```python
from build123d import *

# Parameters (mm, degrees)
F1_DEPTH = 11
F2_D     = 6.3
F3_R     = 5
F4_R     = 2
F5_R     = 1


with BuildPart() as f1:
    # F0 (on Front) → F1 (new body)
    with BuildSketch(Plane.XZ):
        with BuildLine():
            Line((19.1313266688, -1.3), (-19.6425261418, -1.3))
            ThreePointArc((-19.6425261418, -1.3), (-20.5226323435, 3.3504941743), (-24.5, 5.9160797831))
            Line((-24.5, 5.9160797831), (-24.5, 11.5))
            Line((-24.5, 11.5), (-37.5, 11.5))
            Line((-37.5, 11.5), (-37.5, 3.730095943))
            Line((-37.5, 3.730095943), (-26.5, -5.5))
            Line((-26.5, -5.5), (26.5, -5.5))
            ThreePointArc((26.5, -5.5), (37.7208276523, 1.8760988126), (50.5, 6))
            Line((50.5, 6), (50.5, 11.5))
            Line((50.5, 11.5), (38.5, 11.5))
            Line((38.5, 11.5), (28.5361144551, 5.7473479985))
            ThreePointArc((28.5361144551, 5.7473479985), (21.6022101623, 5.2016568881), (19.1313266688, -1.3))
        make_face()
    extrude(amount=-F1_DEPTH)

    # F2 (through all)
    with Locations(Plane.XZ):
        with Locations((25.5, 0), (-25.5, 0)):
            Hole(F2_D / 2)

    # F3
    f3_edges = [f1.edges().sort_by_distance(p)[0] for p in [
        (-24.5, 5.5, 5.91608),
        (-19.642526, 5.5, -1.3),
        (19.131327, 5.5, -1.3),
        (28.536114, 5.5, 5.747348),
        (-37.5, 5.5, 3.730096),
        (-26.5, 5.5, -5.5),
        (26.5, 5.5, -5.5),
        (38.5, 5.5, 11.5),
    ]]
    fillet(f3_edges, radius=F3_R)

    # F4
    f4_edges = [f1.edges().sort_by_distance(p)[0] for p in [
        (-24.5, 5.5, 11.5),
        (-37.5, 5.5, 11.5),
        (50.5, 5.5, 11.5),
        (50.5, 5.5, 6),
    ]]
    fillet(f4_edges, radius=F4_R)

    # F5
    f5_edges = [f1.edges().sort_by_distance(p)[0] for p in [
        (28.771496, 11, 6.278411),
        (-0.264736, 0, -1.3),
    ]]
    fillet(f5_edges, radius=F5_R)


solid = f1.part
```
Geometry check sheet. Reference: the model listing, model coordinates, mm. A direction names the side the tool comes from. Coordinates: 2 decimals unless noted, no trailing zeros. Loops run counter-clockwise (first coordinate to the right, second up) from the corner with the lowest first, then second, coordinate; pieces in that order, holes last. Notation, with made-up numbers: (60.25, -17) - (102.25, -17) arc R15 cw to (102.25, 6) - close; hole circle Ø7 at (44.5, 64.25). An arc over 180 degrees is marked (long way). One line per item, written item: value. Start each with the question number.
(1) Cross-section at B-B on z = 0. Count the separate pieces of the cut face and the enclosed holes in it, plus the area to 3 significant figures.
(2) Mould release check, pull along Z, two halves, no side actions. Record for faces 4 (the cylindrical face through (38.528, 5.563, 11.325)), 5 (the cylindrical face through (22.59, 5.58, -1.21)), 6 (the cylindrical face through (-31.675, 10.699, -0.785)): released by +Z, released by -Z, zero draft, split by the parting line, or undercut.
(3) Material ranges on line 1 (Z direction, x = -6, y = 9); line 2 (X direction, y = 2.25, z = 9); line 3 (Z direction, x = -25.5, y = 3.5), recorded low to high. Write a range as [from, to].
(4) Depth check by flat-ended pin: P1, Ø1.5, axis at x = 33, y = 4.5, coming from the -Z side; P2, Ø10, axis at x = 25.5, z = 0, coming from the -Y side; P3, Ø1.5, axis at y = 5.5, z = 1, coming from the -X side; P4, Ø1, axis at x = 35.5, y = 4, coming from the -Z side. Enter the tip coordinate at first touch or a pass-through.
(5) Cross-section at A-A on y = 2.25. Enter the section's corners in (x, z), plus the area to 3 significant figures.
(6) Tool access check on faces 1 (the cylindrical face through (-23.88, 5.56, 6.81)), 2 (the flat face through (-37.5, 5, 8)), 3 (the cylindrical face through (34.031, 0.285, 8.573)). Record the directions out of +Z, -Z, +X, -X, +Y, -Y that give a thin tool (end or side, any length) a straight path to the whole face; none if there is none.
Results below:
1. separate pieces: 4
1. enclosed holes: 0
1. area: 197 mm2
2. face 4: released by +Z
2. face 5: undercut
2. face 6: released by -Z
3. line 1: z = [-5.5, -1.3]
3. line 2: x = [-37.5, -24.5], [34.17, 50.5]
3. line 3: z = [-5.43, -3.15], [3.15, 11.23]
4. P1: stops at z = -1.18
4. P2: stops at y = 0
4. P3: stops at x = -35.14
4. P4: stops at z = 0.47
5. outline: (-37.5, 6.06) arc R5 ccw to (-35.71, 2.23) - (-27.89, -4.33) arc R5 ccw to (-24.68, -5.5) - (24.68, -5.5) arc R5 ccw to (27.83, -4.38) arc R50 cw to (48.92, 5.69) arc R2 ccw to (50.5, 7.65) - (50.5, 9.5) arc R2 ccw to (48.5, 11.5) - (39.84, 11.5) arc R5 ccw to (37.34, 10.83) - (30.52, 6.89) arc R5 cw to (26.92, 6.34) arc R6.5 ccw to (19.35, 2.09) arc R5 cw to (14.61, -1.3) - (-15.14, -1.3) arc R5 cw to (-19.85, 2.02) arc R6 ccw to (-22.23, 5.03) arc R5 cw to (-24.5, 9.22) - (-24.5, 9.5) arc R2 ccw to (-26.5, 11.5) - (-35.5, 11.5) arc R2 ccw to (-37.5, 9.5) - close; hole circle Ø6.3 at (-25.5, 0); hole circle Ø6.3 at (25.5, 0)
5. area: 603 mm2
6. face 1: +Z, +Y, -Y
6. face 2: +Z, -Z, -X, +Y, -Y
6. face 3: +Z, -Y
